The model under review builds one solid part; all positions refer to its coordinate system, in mm. Round coordinates to 2 decimals unless told otherwise and drop trailing zeros. Write each loop counter-clockwise with the first axis right and the second up, starting at its lowest first coordinate (ties: lowest second). Pieces come first, ordered by that corner, then holes. Notation, with made-up numbers: (26, -15) - (38, -15) arc R14 cw to (38, -3) - close; hole circle Ø9 at (58, -21.5). An arc over 180 degrees is marked (long way). Use one line per item in the form item = value.
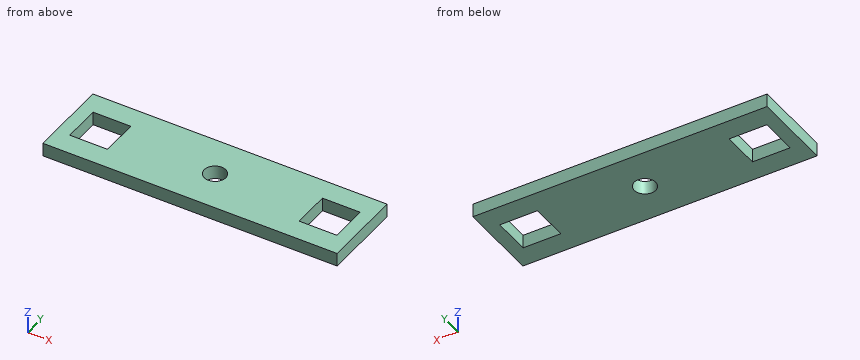
from build123d import *

# Parameters (mm, degrees)
F0_W     = 54.5
F0_H     = 15
F1_DEPTH = 2.5
F3_D     = 4
F4_W     = 7
F4_H     = 7
F5_DEPTH = 2.501


with BuildPart() as f1:
    # F0 (on Top) → F1 (new body)
    with BuildSketch(Plane.XY):
        Rectangle(F0_W, F0_H)
    extrude(amount=F1_DEPTH)

    # F3 (through all)
    with Locations(Plane.XY.offset(2.5)):
        with Locations((0, 0)):
            Hole(F3_D / 2)

    # F4 (on face) → F5 (cut, through all)
    with BuildSketch(Plane.XY.offset(2.5)):
        with Locations((-21.25, 0)):
            Rectangle(F4_W, F4_H)
        with Locations((21.25, 0)):
            Rectangle(F4_W, F4_H)
    extrude(amount=-F5_DEPTH, mode=Mode.SUBTRACT)


solid = f1.part
(1) Add section C-C on z = 0.55. Write out the cut boundary in (x, y).
Geometry results:
outline = (-27.25, -7.5) - (27.25, -7.5) - (27.25, 7.5) - (-27.25, 7.5) - close; hole (-24.75, -3.5) - (-17.75, -3.5) - (-17.75, 3.5) - (-24.75, 3.5) - close; hole circle Ø4 at (0, 0); hole (17.75, -3.5) - (24.75, -3.5) - (24.75, 3.5) - (17.75, 3.5) - close
(2) Add section D-D on x = 0. Write out the cut boundary in (y, z).
Geometry results:
outline = (-7.5, 0) - (-2, 0) - (-2, 2.5) - (-7.5, 2.5) - close; (2, 0) - (7.5, 0) - (7.5, 2.5) - (2, 2.5) - close
(3) Add section B-B on y = 0. Write out the cut boundary in (x, z), then the cut area to 4 significant figures.
Geometry results:
outline = (-27.25, 0) - (-24.75, 0) - (-24.75, 2.5) - (-27.25, 2.5) - close; (-17.75, 0) - (-2, 0) - (-2, 2.5) - (-17.75, 2.5) - close; (2, 0) - (17.75, 0) - (17.75, 2.5) - (2, 2.5) - close; (24.75, 0) - (27.25, 0) - (27.25, 2.5) - (24.75, 2.5) - close
area = 91.25 mm2
(4) Add section A-A on x = 21.5. Write out the cut boundary in (y, z).
Geometry results:
outline = (-7.5, 0) - (-3.5, 0) - (-3.5, 2.5) - (-7.5, 2.5) - close; (3.5, 0) - (7.5, 0) - (7.5, 2.5) - (3.5, 2.5) - close
(5) Insertion check: P1, Ø3.5, axis at x = 0, y = 0, coming from the +Z side. The pin has a flat end and moves straight along its axis. Give the tip position at first contact, or say it passes through.
Geometry results:
P1 = through
(6) To check wall thickness, follow L1, parallel to Y at x = 0, z = 0.8; L2, parallel to Y at x = -18, z = 1.25; L3, parallel to X at y = -1.25, z = 2.35. State the ranges of each line that lie inside material, in increasing order.
Geometry results:
L1 = -7.5 to -2, 2 to 7.5
L2 = -7.5 to -3.5, 3.5 to 7.5
L3 = -27.25 to -24.75, -17.75 to -1.56, 1.56 to 17.75, 24.75 to 27.25
